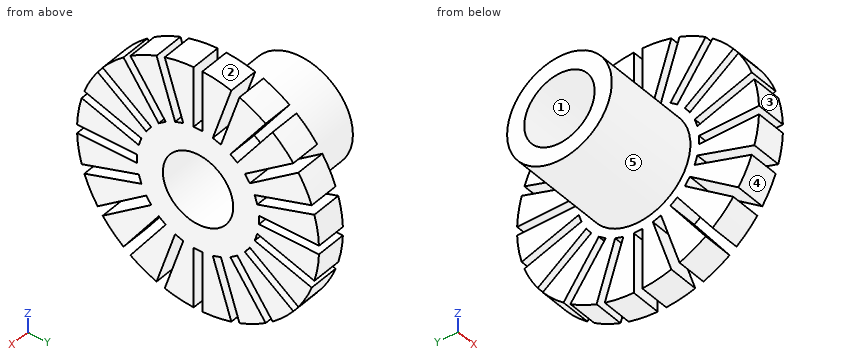
```python
from build123d import *

# Parameters (mm, degrees)
POCKET_DEPTH       = 3.5
POLARPATTERN_COUNT = 20


with BuildPart() as part:
    # Sketch → Revolution (revolve)
    with BuildSketch(Plane.XY):
        Polygon((1.75, 4.1), (1.75, 14.1), (0, 14.1), (-1.75, 14.1), (-1.75, 6.1), (-13.25, 6.1), (-13.25, 4.1), align=None)
    revolve(axis=Axis((0, 0, 0), (1, 0, 0)))

    # Sketch001 (on Face4 of Revolution) → Pocket (cut)
    with BuildSketch(Plane(origin=(-1.75, 0, 0), x_dir=(0, -1, 0), z_dir=(-1, 0, 0))):
        Polygon((-0.5, 15.1), (0.5, 15.1), (0.5, 7.1), (0, 7.1), (-0.5, 7.1), align=None)
    pocket = extrude(amount=-POCKET_DEPTH, mode=Mode.SUBTRACT)

    # PolarPattern: Pocket ×20 about axis
    polarpattern_axis = Axis((-1.75, 0, 0), (-1, 0, 0))
    for i in range(1, POLARPATTERN_COUNT):
        add(pocket.rotate(polarpattern_axis, i * 360 / POLARPATTERN_COUNT), mode=Mode.SUBTRACT)


solid = part.part
```
Part model, mm, in its own coordinate system. Face numbers are marked on the shaded views. A direction names the side the tool comes from. Coordinates: 2 decimals unless noted, no trailing zeros. Order: outer loops, then holes, each group sorted by start corner. A loop starts at its lowest first (then second) coordinate and runs counter-clockwise, first axis right, second up. Notation, with made-up numbers: (-30, 70.5) -> (8, 70.5) arc R27 ccw to (8, 95.5) -> close; hole circle Ø2 at (25, 64.25). An arc over 180 degrees is marked (long way). Put each result on its own line as item: value. Start each with the question number.
(1) Which spindle directions (+Z, -Z, +X, -X, +Y, -Y) get a long thin tool onto all of the face, cutting with end or side? Do the marked faces 4 and 5. Say none if no direction does.
(2) Band-saw the part on C-C (x = -8). Give the cut face in (y, z).
(3) Probe line 1 along Z through (x, y) = (-4.5, 0); line 2 along X through (y, z) = (13.25, -0.75); line 3 along Y through (x, z) = (-9, 2.25). List the from-to ranges inside material, lowest first. Write a range as [from, to].
(4) Mould opens along Y. For the marked faces 1, 2 and 3 say: pulls with the +Y half, pulls with the -Y half, needs draft (parallel to the pull), parting line crosses it, or undercut.
(5) Band-saw the part on A-A (y = 0). Give the cut face in (x, z), then the cut area to 3 significant figures.
(6) Pin check, flat tips, straight feed: pin 1 Ø1 at (x, y) = (1, -10) entering from -Z; pin 2 Ø1 at (x, z) = (0, 10.5) entering from -Y; pin 3 Ø1.8 at (x, z) = (-0.5, -11) entering from +Y; pin 4 Ø8 at (y, z) = (0, 8.5) entering from -X. Stop position of each tip, or through.
Determined:
1. face 4: -Z, +X, -X, -Y
1. face 5: -X
2. outline: circle Ø12.2 at (0, 0); hole circle Ø8.2 at (0, 0)
3. line 1: z = [-6.1, -4.1], [4.1, 6.1]
3. line 2: x = [-1.75, 1.75]
3. line 3: y = [-5.67, -3.43], [3.43, 5.67]
4. face 1: undercut
4. face 2: pulls with the +Y half
4. face 3: pulls with the -Y half
5. outline: (-13.25, -6.1) -> (-1.75, -6.1) -> (-1.75, -7.1) -> (1.75, -7.1) -> (1.75, -4.1) -> (-13.25, -4.1) -> close; (-13.25, 4.1) -> (1.75, 4.1) -> (1.75, 7.1) -> (-1.75, 7.1) -> (-1.75, 6.1) -> (-13.25, 6.1) -> close
5. area: 67.0 mm²
6. pin 1: stops at z = -10.42
6. pin 2: stops at y = -9.94
6. pin 3: stops at y = 9.84
6. pin 4: stops at x = -13.25
